Can you work these out from the model? Positions are in its coordinate system, mm. A direction names the side the tool comes from. Round coordinates to 2 decimals unless told otherwise and drop trailing zeros. Order: outer loops, then holes, each group sorted by start corner. A loop starts at its lowest first (then second) coordinate and runs counter-clockwise, first axis right, second up. Notation, with made-up numbers: (-38, -33) -> (-31, -33) arc R27 ccw to (-31, -9) -> close; hole circle Ø7 at (74.25, -10.5). An arc over 180 degrees is marked (long way). One line per item, written item: value.
```python
from build123d import *

# Parameters (mm, degrees)
REVOLUTION_ANGLE = 60
SKETCH001_R      = 13
PAD_DEPTH        = 4


with BuildPart() as part:
    # Sketch → Revolution (revolve)
    with BuildSketch(Plane.XY):
        Polygon((-26, 25), (26, 25), (26, 29), (23, 29), (23, 28), (15, 28), (15, 29), (-15, 29), (-15, 28), (-23, 28), (-23, 29), (-26, 29), align=None)
    revolve(axis=Axis((0, 0, 0), (1, 0, 0)), revolution_arc=REVOLUTION_ANGLE)

    # Sketch001 (on DatumPlane) → Pad (new body)
    with BuildSketch(Plane(origin=(0.333333, 24.166667, 8.371579), x_dir=(1, 0, 0), z_dir=(0, -0.866025, -0.5))):
        with Locations((-0.333333, 4.833333)):
            Circle(SKETCH001_R)
    extrude(amount=-PAD_DEPTH)


solid = part.part
```
Q1. We'd pull the mould along Y, two halves only. Please class faces 4 (the face through (-0.182, 25.123, 14.715)), 5 (the face through (-0.364, 13.514, 23.407)), 6 (the face through (-23, 24.3, 14.5)), 7 (the face through (-2.818, 30.465, 2.935)): released by +Y, released by -Y, zero draft, split by the parting line, or undercut.
Answers below:
face 4: released by +Y
face 5: released by -Y
face 6: zero draft
face 7: undercut
Q2. I want a section at B-B on x = -12.5. List the corners of the cut face in (y, z) for me.
Answers below:
outline: (12.5, 21.65) arc R25 cw to (25, 0) -> (29, 0) arc R29 ccw to (26.71, 11.3) -> (27, 11.47) -> (23.43, 17.65) -> (23.14, 17.48) arc R29 ccw to (14.5, 25.11) -> close
Q3. I want a section at A-A on x = -4. List the corners of the cut face in (y, z) for me.
Answers below:
outline: (12.5, 21.65) arc R25 cw to (25, 0) -> (29, 0) arc R29 ccw to (28.9, 2.4) -> (31.4, 3.85) -> (19.03, 25.27) -> (16.53, 23.83) arc R29 ccw to (14.5, 25.11) -> close
Q4. Will these pins go through, and if not, where does the flat tip stop? pin 1 Ø10 at (x, z) = (8.5, 19) entering from +Y; pin 2 Ø8 at (x, z) = (0.5, 13) entering from +Y; pin 3 Ø12 at (x, z) = (13, 10) entering from -Y; pin 4 Ø12 at (x, z) = (-6, 4) entering from +Y.
Answers below:
pin 1: y = 25.54
pin 2: y = 28.42
pin 3: y = 19.21
pin 4: y = 31.71
Q5. I want a section at C-C on x = 18. List the corners of the cut face in (y, z) for me.
Answers below:
outline: (12.5, 21.65) arc R25 cw to (25, 0) -> (28, 0) arc R28 ccw to (14, 24.25) -> close
Q6. On a 3-axis mill with a long thin cutter (end or side, diameter ignored), from which of +Z, -Z, +X, -X, +Y, -Y can I reach the whole of each face in a straight line? I mean faces 1 (the face through (18.94, 24.35, 13.82)), 2 (the face through (24.48, 25.22, 14.32)), 3 (the face through (-24.52, 25.22, 14.32)). Say none if no direction works.
Answers below:
face 1: +Z, +Y
face 2: +Z, +X, +Y
face 3: +Z, -X, +Y
Q7. Please list where these lines run through material, in increasing order: line 1 along X through (y, z) = (19.25, 21.5); line 2 along Y through (x, z) = (17, 12); line 3 along Z through (x, y) = (15.5, 23).
Answers below:
line 1: -26 to -23, -15 to 15, 23 to 26
line 2: 21.93 to 25.3
line 3: 9.8 to 15.97
